from build123d import *

# Parameters (mm, degrees)
SKETCH1_R      = 4.5
EXTRUDE1_DEPTH = 6.35


with BuildPart() as part:
    # Sketch1 → Extrude1 (new body)
    with BuildSketch(Plane(origin=(0, 0, 0), x_dir=(1, 0, 0), z_dir=(0, 1, 0))):
        with BuildLine():
            Line((32.812063874, 55.953109441), (55.379571692, 55.997622064))
            ThreePointArc((55.379571692, 55.997622064), (57.288458974, 56.688173959), (58.320639688, 58.436120054))
            ThreePointArc((58.320639688, 58.436120054), (74.0236038, 68.667854555), (83.630875665, 52.575253766))
            ThreePointArc((83.630875665, 52.575253766), (83.636046743, 50.974550497), (84.463614261, 49.604364488))
            ThreePointArc((84.463614261, 49.604364488), (95.435770873, 32.172746021), (96.641280568, 11.610735189))
            ThreePointArc((96.641280568, 11.610735189), (96.705732474, 10.194548777), (97.413259954, 8.966077015))
            ThreePointArc((97.413259954, 8.966077015), (96.34909056, -9.964571582), (77.524483139, -7.698282048))
            ThreePointArc((77.524483139, -7.698282048), (76.978786155, -7.130320059), (76.304071652, -6.723962634))
            ThreePointArc((76.304071652, -6.723962634), (44, 0), (11.695928348, -6.723962634))
            ThreePointArc((11.695928348, -6.723962634), (11.021213845, -7.130320059), (10.475516861, -7.698282048))
            ThreePointArc((10.475516861, -7.698282048), (-8.364205722, -9.951887391), (-9.385998192, 8.994611606))
            ThreePointArc((-9.385998192, 8.994611606), (-8.674953739, 10.220222023), (-8.60571551, 11.635464468))
            ThreePointArc((-8.60571551, 11.635464468), (-7.328831083, 32.189532865), (3.700447598, 49.58077127))
            ThreePointArc((3.700447598, 49.58077127), (4.532944762, 50.949409073), (4.542457699, 52.551323698))
            ThreePointArc((4.542457699, 52.551323698), (14.169725803, 68.615280401), (29.859544881, 58.389598348))
            ThreePointArc((29.859544881, 58.389598348), (30.896689666, 56.63923798), (32.812063874, 55.953109441))
        make_face()
        with Locations(Location((17.090937333, 55.947742234, 0), (0, 0, 270))):  # turned: the seam where the file's is
            Circle(SKETCH1_R, mode=Mode.SUBTRACT)
        with Locations(Location((71.090909091, 56.002969963, 0), (0, 0, 270))):  # turned: the seam where the file's is
            Circle(SKETCH1_R, mode=Mode.SUBTRACT)
        with Locations(Location((0, 0, 0), (0, 0, 270))):  # turned: the seam where the file's is
            Circle(SKETCH1_R, mode=Mode.SUBTRACT)
        with Locations(Location((88, 0, 0), (0, 0, 270))):  # turned: the seam where the file's is
            Circle(SKETCH1_R, mode=Mode.SUBTRACT)
    extrude(amount=EXTRUDE1_DEPTH)


solid = part.part
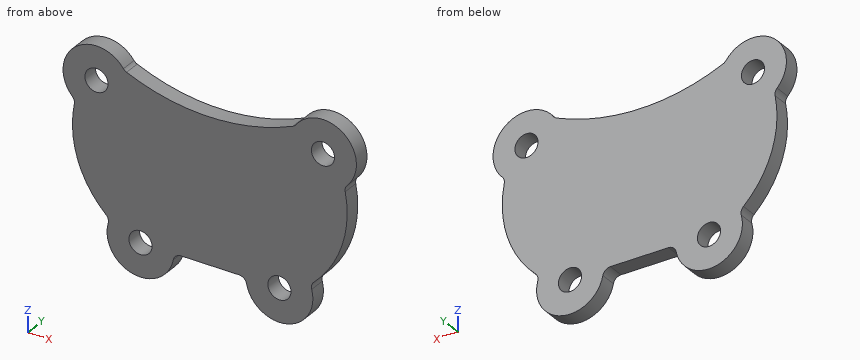
Source: CAD feature listing. Evaluate the final solid. Frame: model axes, mm. Give positions to 0.01 mm unless a question says otherwise; leave off trailing zeros. Write each loop counter-clockwise with the first axis right and the second up, starting at its lowest first coordinate (ties: lowest second). Pieces come first, ordered by that corner, then holes. Notation, with made-up numbers: (31, 43.5) -> (76, 43.5) arc R20 cw to (76, 79.5) -> close; hole circle Ø2 at (-18.5, -11.5). An arc over 180 degrees is marked (long way). Return JSON: item names as keys, results as strings. Group by question number.
1. Pin query (flat end, axial travel): pin 1 Ø5 at (x, z) = (28, -29) entering from -Y; pin 2 Ø1 at (y, z) = (4, -4.5) entering from -X; pin 3 Ø3 at (x, y) = (35.5, 1.5) entering from -Z; pin 4 Ø5.5 at (x, z) = (71.09, -56) entering from +Y. Return the tip coordinate at first contact, or that it passes through.
2. Section A-A, the plane x = 0. Output: boundary loops of the cut face in (y, z).
3. Section C-C, the plane x = 88. Output: boundary loops of the cut face in (y, z), then the cut area to 3 significant figures.
4. Material intervals for line 1 (X direction, y = 2, z = -3); line 2 (X direction, y = 1.5, z = -57); line 3 (Z direction, x = 19.5, y = 0.75), sorted ascending. Write a range as from..to.
5. Section B-B, the plane z = -23.5. Output: boundary loops of the cut face in (x, y).
6. Section D-D, the plane x = 49. Output: boundary loops of the cut face in (y, z).
Determined:
{
 "1": {"pin 1": "stops at y = 0", "pin 2": "stops at x = -12.37", "pin 3": "stops at z = -55.96", "pin 4": "passes through"},
 "2": {"outline": "(0, -45.62) -> (6.35, -45.62) -> (6.35, -4.5) -> (0, -4.5) -> close; (0, 4.5) -> (6.35, 4.5) -> (6.35, 13) -> (0, 13) -> close"},
 "3": {"outline": "(0, -45.81) -> (6.35, -45.81) -> (6.35, -4.5) -> (0, -4.5) -> close; (0, 4.5) -> (6.35, 4.5) -> (6.35, 13) -> (0, 13) -> close", "area": "316 mm2"},
 "4": {"line 1": "x = -12.65..-3.35, 3.35..84.65, 91.35..100.65", "line 2": "x = 4.13..12.72, 21.47..30.53, 57.61..66.7, 75.48..84.05", "line 3": "z = -68.72..-59.75, -52.15..3.8"},
 "5": {"outline": "(-9.15, 0) -> (97.22, 0) -> (97.22, 6.35) -> (-9.15, 6.35) -> close"},
 "6": {"outline": "(0, -55.99) -> (6.35, -55.99) -> (6.35, 0.15) -> (0, 0.15) -> close"}
}
